Here's how the part is built. I have some questions about the finished solid (model axes, mm). A direction names the side the tool comes from. Coordinates: 2 decimals unless noted, no trailing zeros. Order: outer loops, then holes, each group sorted by start corner. A loop starts at its lowest first (then second) coordinate and runs counter-clockwise, first axis right, second up.
```python
from build123d import *

# Parameters (mm, degrees)
F1_DEPTH = 1


with BuildPart() as f1:
    # F0 (on Front) → F1 (new body)
    with BuildSketch(Plane.XZ):
        with BuildLine():
            ThreePointArc((0.5134190636, 20.3306143382), (4.1745945423, 22.1487100844), (5.6526372145, 25.9598867907))
            ThreePointArc((5.6526372145, 25.9598867907), (-3.8111767063, 30.134481333), (-0.5134190636, 20.3306143382))
            Line((-0.5134190636, 20.3306143382), (0.5134190636, 20.3306143382))
        make_face()
        with BuildLine():
            Line((0.5134190636, 20.3306143382), (-0.5134190636, 20.3306143382))
            ThreePointArc((-0.5134190636, 20.3306143382), (0, 20.3072495762), (0.5134190636, 20.3306143382))
        make_face()
        with BuildLine():
            ThreePointArc((0.5134190636, 20.3306143382), (0, 20.3072495762), (-0.5134190636, 20.3306143382))
            Line((-0.5134190636, 20.3306143382), (-11.4882850616, 20.3306143382))
            Line((-11.4882850616, 20.3306143382), (-11.4882850616, 0))
            Line((-11.4882850616, 0), (-4.4247405394, 0))
            Line((-4.4247405394, 0), (-4.4247405394, 7.7945953777))
            Line((-4.4247405394, 7.7945953777), (-2.0671913816, 0))
            Line((-2.0671913816, 0), (2.0671913816, 0))
            Line((2.0671913816, 0), (4.4247405394, 7.7945953777))
            Line((4.4247405394, 7.7945953777), (4.4247405394, 0.0472759202))
            Line((4.4247405394, 0.0472759202), (11.4850704372, 0.0472759202))
            Line((11.4850704372, 0.0472759202), (11.4850704372, 20.3306143382))
            Line((11.4850704372, 20.3306143382), (0.5134190636, 20.3306143382))
        make_face()
    extrude(amount=F1_DEPTH)


solid = f1.part
```
Q1. I need wall thicknesses on L1, parallel to X at y = -0.8, z = 6; L2, parallel to X at y = -0.15, z = 2; L3, parallel to Z at x = 10.5, y = -0.3. Which ranges of each line are inside material? Lowest first, please.
Q2. If we section it at C-C on x = -4: Write out the boundary of the cut face in (y, z), then the cut area to 3 significant figures.
Q3. If we section it at A-A on z = 5: Write out the boundary of the cut face in (x, y), then the cut area to 3 significant figures.
Q4. Will these pins go through, and if not, where does the flat tip stop? pin 1 (0.5 mm diameter, centred on x = -4.5, y = -0.5, fed in from +Z); pin 2 (12 mm diameter, centred on x = -5, z = 5, fed in from +Y).
Q5. We'd pull the mould along Z, two halves only. Please class faces 1 (the flat face through (6.1, -0.5, 20.331)), 2 (the flat face through (-8, -0.5, 0)), 3 (the flat face through (0, -1, 13)): pulls with the +Z half, pulls with the -Z half, needs draft (parallel to the pull), parting line crosses it, or undercut.
Q6. For faces 4 (the flat face through (7.9, -0.5, 0.047)), 5 (the flat face through (-3.26, -0.49, 3.95)), 6 (the flat face through (0, -0.5, 0)), which set-ups out of +Z, -Z, +X, -X, +Y, -Y let a thin tool reach every point of the face, with its end or its side?
Q7. If we section it at D-D on z = 24: Write out the boundary of the cut face in (x, y), then the cut area to 3 significant figures.
Q8. If we section it at B-B on y = -0.75: Write out the boundary of the cut face in (x, z), then the cut area to 3 significant figures.
Reply:
1. L1: x = -11.49 to -4.42, -3.88 to 3.88, 4.42 to 11.49
1. L2: x = -11.49 to -4.42, -2.67 to 2.67, 4.42 to 11.49
1. L3: z = 0.05 to 20.33
2. outline: (-1, 6.39) - (0, 6.39) - (0, 20.33) - (-1, 20.33) - close; (-1, 21.97) - (0, 21.97) - (0, 29.95) - (-1, 29.95) - close
2. area: 21.9 mm2
3. outline: (-11.49, -1) - (-4.42, -1) - (-4.42, 0) - (-11.49, 0) - close; (-3.58, -1) - (3.58, -1) - (3.58, 0) - (-3.58, 0) - close; (4.42, -1) - (11.49, -1) - (11.49, 0) - (4.42, 0) - close
3. area: 21.3 mm2
4. pin 1: stops at z = 29.69
4. pin 2: stops at y = 0
5. face 1: undercut
5. face 2: pulls with the -Z half
5. face 3: needs draft
6. face 4: -Z, +X, +Y, -Y
6. face 5: -Z, +Y, -Y
6. face 6: -Z, +X, -X, +Y, -Y
7. outline: (-5.3, -1) - (5.3, -1) - (5.3, 0) - (-5.3, 0) - close
7. area: 10.6 mm2
8. outline: (-11.49, 0) - (-4.42, 0) - (-4.42, 7.79) - (-2.07, 0) - (2.07, 0) - (4.42, 7.79) - (4.42, 0.05) - (11.49, 0.05) - (11.49, 20.33) - (0.51, 20.33) arc R5.65 ccw (long way) to (-0.51, 20.33) - (-11.49, 20.33) - close
8. area: 549 mm2
